Geometry: final body of the model. Coordinates: model frame, mm. A direction names the side the tool comes from. Round coordinates to 2 decimals unless told otherwise and drop trailing zeros. Loops run counter-clockwise (first coordinate to the right, second up) from the corner with the lowest first, then second, coordinate; pieces in that order, holes last. Notation, with made-up numbers: M -33.75,-4.75 L 2.25,-4.75 A18 ccw 2.25,22.25 Z; hole C -21,69.5 d11. An arc over 180 degrees is marked long. Return JSON: item names as keys, results as strings.
from build123d import *


with BuildPart() as f1:
    # F0 (on Front) → F1 (revolve)
    with BuildSketch(Plane.XZ):
        Polygon((23.9, -34.5), (19.503332, -34.5), (15, -42.3), (15, -47.55), (13.4, -47.55), (13.4, -50.3), (16.5, -50.3), (16.5, -42.3), (26.05, -42.3), (26.05, -41), (25.05, -41), (25.05, -40), (24.55, -39.5), (23.9, -39.5), (23.9, -38.5), (22.626104, -38.5), (23.9, -35), align=None)
    revolve(axis=Axis((0, 0, -9.429786), (0, 0, -1)))


solid = f1.part
Q1. Pull-direction query (Z, two-part tool) for faces 4 (the conical face through (21.657, -6.82, -38.281)), 5 (the cylindrical face through (-13.387, -0.589, -48.944)), 6 (the flat face through (0, -14, -50.3)), 7 (the flat face through (-14, 18, -38.5)); classes: pulls with the +Z half, pulls with the -Z half, needs draft (parallel to the pull), parting line crosses it, or undercut.
Determined:
{"face 4": "undercut", "face 5": "needs draft", "face 6": "pulls with the -Z half", "face 7": "undercut"}
Q2. Reachability of faces 1 (the flat face through (-20, 0, -34.5)), 2 (the cylindrical face through (15.24, 6.32, -46.24)), 3 (the cylindrical face through (12.85, -20.15, -38.99)) from +Z, -Z, +X, -X, +Y, -Y: full face, straight path, thin tool, end or side. Return the list, or none.
Determined:
{"face 1": "+Z, +X, -X, +Y, -Y", "face 2": "-Z", "face 3": "+Z"}
Q3. Section query C-C (z = -46). Output: boundary loops of the cut face in (x, y), plus the area to 3 significant figures.
Determined:
{"outline": "C 0,0 d33; hole C 0,0 d30", "area": "148 mm^2"}
Q4. Pin query (flat end, axial travel): pin 1 (4 mm diameter, centred on x = 4, y = 20.5, fed in from -Z); pin 2 (6 mm diameter, centred on y = -6, z = -45, fed in from +X); pin 3 (1 mm diameter, centred on x = 1, z = -43, fed in from +Y); pin 4 (21.5 mm diameter, centred on x = 0, y = 0, fed in from -Z). Return the tip coordinate at first contact, or that it passes through.
Determined:
{"pin 1": "stops at z = -42.3", "pin 2": "stops at x = 25.62", "pin 3": "stops at y = 16.49", "pin 4": "passes through"}
Q5. Material intervals for L1, parallel to Y at x = 0, z = -49.25; L2, parallel to X at y = 0, z = -45.85, sorted ascending.
Determined:
{"L1": "y = -16.5 to -13.4, 13.4 to 16.5", "L2": "x = -16.5 to -15, 15 to 16.5"}
